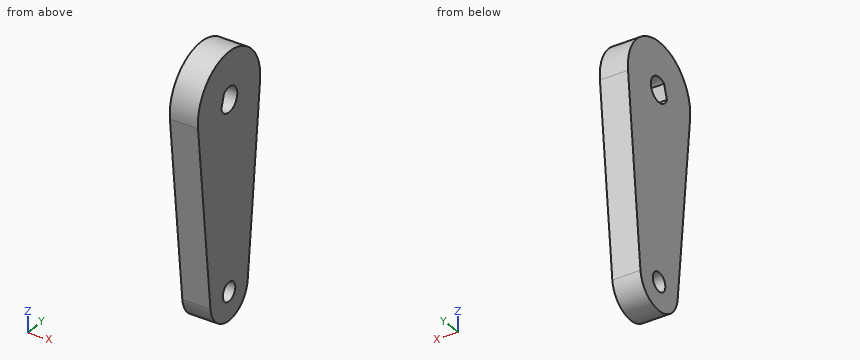
```python
from build123d import *

# Parameters (mm, degrees)
SKETCH1_R                = 10
SKETCH1_R_2              = 6
BOSS_EXTRUDE1_DEPTH      = 3
BOSS_EXTRUDE1_DEPTH_BACK = 3
SKETCH2_R                = 2
CUT_EXTRUDE1_DEPTH       = 4
CUT_EXTRUDE1_DEPTH_BACK  = 4
CUT_EXTRUDE2_DEPTH       = 10


with BuildPart() as part:
    # Sketch1 → Boss-Extrude1 (new body, two sides)
    with BuildSketch(Plane(origin=(0, 0, 0), x_dir=(0, 0, -1), z_dir=(1, 0, 0))) as boss_extrude1_sk:
        Circle(SKETCH1_R)
        with BuildLine():
            Line((1, -9.949874371), (40.6, -5.969924623))
            ThreePointArc((40.6, -5.969924623), (34, 0), (40.6, 5.969924623))
            Line((40.6, 5.969924623), (1, 9.949874371))
            ThreePointArc((1, 9.949874371), (7.416198487, 6.708203932), (10, 0))
            ThreePointArc((10, 0), (7.416198487, -6.708203933), (1, -9.949874371))
        make_face()
        with Locations((40, 0)):
            Circle(SKETCH1_R_2)
    extrude(amount=BOSS_EXTRUDE1_DEPTH)
    extrude(boss_extrude1_sk.sketch, amount=-BOSS_EXTRUDE1_DEPTH_BACK)

    # Sketch2 → Cut-Extrude1 (cut, two sides)
    with BuildSketch(Plane(origin=(0, 0, 0), x_dir=(0, 0, -1), z_dir=(1, 0, 0))) as cut_extrude1_sk:
        with Locations((40, 0)):
            Circle(SKETCH2_R)
    extrude(amount=CUT_EXTRUDE1_DEPTH, mode=Mode.SUBTRACT)
    extrude(cut_extrude1_sk.sketch, amount=-CUT_EXTRUDE1_DEPTH_BACK, mode=Mode.SUBTRACT)

    # Sketch3 → Cut-Extrude2 (cut)
    with BuildSketch(Plane(origin=(3, 0, 0), x_dir=(0, 0, -1), z_dir=(1, 0, 0))):
        with BuildLine():
            Line((-2.09135741, -1.616067196), (0.829813276, -2.509354285))
            ThreePointArc((0.829813276, -2.509354285), (0.772893172, 2.527466151), (-2.09135741, -1.616067196))
        make_face()
    extrude(amount=-CUT_EXTRUDE2_DEPTH, mode=Mode.SUBTRACT)


solid = part.part
```
Here's how the part is built. I have some questions about the finished solid (model axes, mm). Round coordinates to 2 decimals unless told otherwise and drop trailing zeros. Order: outer loops, then holes, each group sorted by start corner. A loop starts at its lowest first (then second) coordinate and runs counter-clockwise, first axis right, second up. Notation, with made-up numbers: M 59.25,79 L 101.25,79 A14 ccw 101.25,85 Z; hole C -40,6.25 d7. An arc over 180 degrees is marked long. Answer in a Markdown table with one row per item.
Item 1: If I drill on L1, parallel to Z at x = 2.5, y = 1.25; L2, parallel to Y at x = 0.15, z = 1; L3, parallel to Y at x = -0.4, z = -40, over which ranges is the centre line in solid material (lowest first)? Write a range as from..to.
A:
| item | result |
|---|---|
| L1 | z = -45.87..-41.56, -38.44..-2.33, 2.33..9.92 |
| L2 | y = -9.95..-1.95, 2.45..9.95 |
| L3 | y = -6.03..-2, 2..6.03 |
Item 2: Imagine slicing it at B-B, the plane x = -1.7. Write out the boundary of the cut face in (y, z), and give its area (3 significant figures).
A:
| item | result |
|---|---|
| outline | M -9.95,-1 L -5.97,-40.6 A6 ccw 5.97,-40.6 L 9.95,-1 A10 ccw long Z; hole M -2.51,-0.83 A2.64 ccw long -1.62,2.09 Z; hole C 0,-40 d4 |
| area | 823 mm2 |
Item 3: Imagine slicing it at A-A, the plane y = 0. Write out the boundary of the cut face in (x, z).
A:
| item | result |
|---|---|
| outline | M -3,-46 L 3,-46 L 3,-42 L -3,-42 Z; M -3,-38 L 3,-38 L 3,-2.64 L -3,-2.64 Z; M -3,2.64 L 3,2.64 L 3,10 L -3,10 Z |
Item 4: Imagine slicing it at D-D, the plane z = 0. Write out the boundary of the cut face in (x, y), and give its area (3 significant figures).
A:
| item | result |
|---|---|
| outline | M -3,-10 L 3,-10 L 3,-2.26 L -3,-2.26 Z; M -3,2.64 L 3,2.64 L 3,10 L -3,10 Z |
| area | 90.6 mm2 |
Item 5: Imagine slicing it at C-C, the plane z = -40. Write out the boundary of the cut face in (x, y), and give its area (3 significant figures).
A:
| item | result |
|---|---|
| outline | M -3,-6.03 L 3,-6.03 L 3,-2 L -3,-2 Z; M -3,2 L 3,2 L 3,6.03 L -3,6.03 Z |
| area | 48.4 mm2 |
Item 6: I'm going to push flat-ended pins straight in: pin 1 (5 mm diameter, centred on y = 0, z = 0, fed in from -X); pin 2 (3 mm diameter, centred on x = 2.5, z = -20, fed in from +Y). Where does each tip first touch, or does it pass through?
A:
| item | result |
|---|---|
| pin 1 | stops at x = -3 |
| pin 2 | stops at y = 8.19 |
